```python
from build123d import *

# Parameters (mm, degrees)
F0_R     = 5
F1_DEPTH = 600


with BuildPart() as f1:
    # F0 (on Top) → F1 (new body)
    with BuildSketch(Plane.XY):
        with BuildLine():
            Line((30, 6), (30, 30))
            Line((30, 30), (6, 30))
            Line((6, 30), (6, 24))
            Line((6, 24), (10, 24))
            Line((10, 24), (10, 14))
            ThreePointArc((10, 14), (5.176381, 12.001992), (0, 11.320508))
            Line((0, 11.320508), (0, 6))
            ThreePointArc((0, 6), (4.242641, 4.242641), (6, 0))
            ThreePointArc((6, 0), (4.242641, -4.242641), (0, -6))
            Line((0, -6), (0, -11.320508))
            ThreePointArc((0, -11.320508), (5.176381, -12.001992), (10, -14))
            Line((10, -14), (10, -24))
            Line((10, -24), (6, -24))
            Line((6, -24), (6, -30))
            Line((6, -30), (30, -30))
            Line((30, -30), (30, -6))
            Line((30, -6), (24, -6))
            Line((24, -6), (24, -10))
            Line((24, -10), (14, -10))
            ThreePointArc((14, -10), (11.132038, 0), (14, 10))
            Line((14, 10), (24, 10))
            Line((24, 10), (24, 6))
            Line((24, 6), (30, 6))
        make_face()
        with Locations((20, -20)):
            Circle(F0_R, mode=Mode.SUBTRACT)
        with Locations((20, 20)):
            Circle(F0_R, mode=Mode.SUBTRACT)
        with BuildLine():
            Line((0, 6), (0, 11.320508))
            ThreePointArc((0, 11.320508), (-5.176381, 12.001992), (-10, 14))
            Line((-10, 14), (-10, 24))
            Line((-10, 24), (-6, 24))
            Line((-6, 24), (-6, 30))
            Line((-6, 30), (-30, 30))
            Line((-30, 30), (-30, 6))
            Line((-30, 6), (-24, 6))
            Line((-24, 6), (-24, 10))
            Line((-24, 10), (-14, 10))
            ThreePointArc((-14, 10), (-11.132038, 0), (-14, -10))
            Line((-14, -10), (-24, -10))
            Line((-24, -10), (-24, -6))
            Line((-24, -6), (-30, -6))
            Line((-30, -6), (-30, -30))
            Line((-30, -30), (-6, -30))
            Line((-6, -30), (-6, -24))
            Line((-6, -24), (-10, -24))
            Line((-10, -24), (-10, -14))
            ThreePointArc((-10, -14), (-5.176381, -12.001992), (0, -11.320508))
            Line((0, -11.320508), (0, -6))
            ThreePointArc((0, -6), (-6, 0), (0, 6))
        make_face()
        with Locations((-20, -20)):
            Circle(F0_R, mode=Mode.SUBTRACT)
        with Locations((-20, 20)):
            Circle(F0_R, mode=Mode.SUBTRACT)
    extrude(amount=F1_DEPTH)


solid = f1.part
```
Verification items for the finished model (mm, model axes). A direction names the side the tool comes from. Round coordinates to 2 decimals unless told otherwise and drop trailing zeros. Answer as a JSON object with one key per item and string values. Group by question number.
Q1. Section check A-A, the plane z = 454. Give the number of separate pieces and of enclosed holes in the cut face, plus the area to 3 significant figures.
Q2. Mould release check, pull along Y, two halves, no side actions. Record for faces 3 (the flat face through (0, 7, 600)), 4 (the flat face through (-18, 30, 296)), 5 (the flat face through (-19, 10, 296)): released by +Y, released by -Y, zero draft, split by the parting line, or undercut.
Q3. Go/stop test with flat-tipped pins: pin 1 Ø13 at (x, y) = (20, 20) entering from +Z; pin 2 Ø6 at (x, y) = (-21, 19) entering from +Z. Record where each tip stops, or that it passes through.
Q4. Thickness scan on line 1 (Y direction, x = 20, z = 475); line 2 (X direction, y = -14, z = 541); line 3 (X direction, y = -26, z = 161.5). Record the ranges inside material, lowest first.
Q5. Tool access check on faces 1 (the flat face through (30, -18, 296)), 2 (the flat face through (10, 19, 296)). Record the directions out of +Z, -Z, +X, -X, +Y, -Y that give a thin tool (end or side, any length) a straight path to the whole face; none if there is none.
Found:
{
 "1": {"separate pieces": "1", "enclosed holes": "5", "area": "1,930 mm^2"},
 "2": {"face 3": "zero draft", "face 4": "released by +Y", "face 5": "undercut"},
 "3": {"pin 1": "stops at z = 600", "pin 2": "passes through"},
 "4": {"line 1": "y = -30 to -25, -15 to -10, 10 to 15, 25 to 30", "line 2": "x = -30 to -10, 10 to 30", "line 3": "x = -30 to -6, 6 to 30"},
 "5": {"face 1": "+Z, -Z, +X, +Y, -Y", "face 2": "+Z, -Z"}
}
